from build123d import *

# Parameters (mm, degrees)
F2_R = 50
F1_W = 50
F1_H = 50
F4_T = 2.5


# Not quite as in the source:
# - a shell that OpenCascade refuses in one call is made with other operations: the cavity is built on its own and cut out


with BuildPart() as f3:
    # F2 (on offset) → F3 section 0
    with BuildSketch(Plane.XY.offset(150)):
        Circle(F2_R)
    # F1 (on Top) → F3 section 1
    with BuildSketch(Plane.XY):
        Rectangle(F1_W, F1_H)
    loft()

    # F4: shell of thickness 2.5, made by hand


with BuildPart() as f4_core1:
    # F4_t2: copy of F3
    add(f3.part)

    # the walls: a layer under each face that stays
    f4_faces = [f4_core1.faces().sort_by_distance(p)[0] for p in [
        (35.5969883078, 15.8170858071, 75),
        (0, 37.4999999981, 75),
        (-37.4999999981, 0, 75),
        (0, -37.4999999981, 75),
        (35.5969883078, -15.8170858071, 75),
        (0, 0, 0),
    ]]
    thicken(f4_faces, amount=-F4_T, mode=Mode.SUBTRACT)


with BuildPart() as f3_1:
    add(f3.part)

    # what is left inside the walls is the cavity
    f4_cavity = [f4_core1.part.solids().sort_by_distance(p)[0] for p in [
        (-39.265085, 0, 100.949484),
    ]]
    add(f4_cavity, mode=Mode.SUBTRACT)


solid = f3_1.part
The model under review builds one solid part; all positions refer to its coordinate system, in mm. Coordinates: 2 decimals unless noted, no trailing zeros. Answer as a JSON object with one key per item and string values. Group by question number.
1. Mouldability with a two-part tool opening along X and no side actions: class faces 1 (the face through (0, -1, 0)), 2 (the face through (0, -1, 2.5)) as pulls with the +X half, pulls with the -X half, needs draft (parallel to the pull), parting line crosses it, or undercut.
2. Clearance check with flat-ended pins moving along their axes: pin 1 Ø1 at (y, z) = (-26, 25.5) entering from +X; pin 2 Ø4 at (x, z) = (-35.5, 126) entering from +Y; pin 3 Ø2 at (y, z) = (-32, 85) entering from +X. State where each tip first meets the part, or that it passes through.
3. To check wall thickness, follow probe 1 along X at (y, z) = (11, 59.5); probe 2 along X at (y, z) = (34, 124.5); probe 3 along Z at (x, y) = (-17, 10.5). State the ranges of each line that lie inside material, in increasing order.
Findings:
{
 "1": {"face 1": "needs draft", "face 2": "undercut"},
 "2": {"pin 1": "x = 27", "pin 2": "y = 33.89", "pin 3": "x = 30.65"},
 "3": {"probe 1": "-34.12 to -31.57, 31.57 to 34.12", "probe 2": "-33.11 to -28.98, 28.98 to 33.11", "probe 3": "0 to 2.5"}
}
